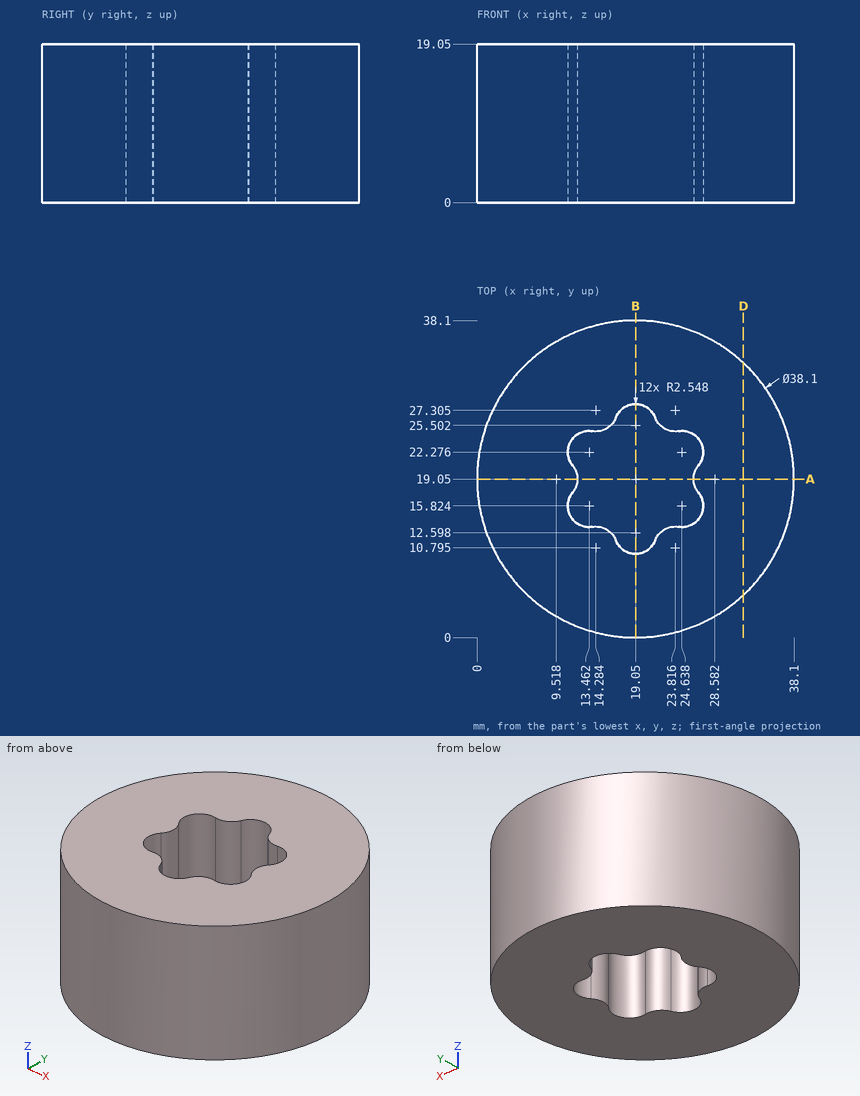
Input: dimensioned drawing with shaded views. Units: mm. Origin: part minimum x, y, z. Round coordinates to 2 decimals unless told otherwise and drop trailing zeros. Order: outer loops, then holes, each group sorted by start corner. A loop starts at its lowest first (then second) coordinate and runs counter-clockwise, first axis right, second up. Notation, with made-up numbers: (55, 76) -> (91, 76) arc R17 cw to (91, 96) -> close; hole circle Ø3 at (76, 78.25). An arc over 180 degrees is marked (long way). Put each result on its own line as item: value. Start each with the question number.
Q1. Section D-D on x = 32. Return the cut outline in (y, z), and give its area (3 significant figures).
Q2. First-contact query: pin 1 (1 mm diameter, centred on x = 30.5, z = 9.5, fed in from -Y); pin 2 (2 mm diameter, centred on x = 21, z = 11, fed in from -Y); pin 3 (8 mm diameter, centred on y = 33, z = 12.5, fed in from -X) (1 decimal); pin 4 (8 mm diameter, centred on x = 26.5, y = 17.5, fed in from +Z). Flat tips, straight axial feed; report the tip coordinate or a pass-through.
Q3. Line query: probe 1 along X at (y, z) = (19, 13.25) (1 decimal); probe 2 along Y at (x, z) = (24, 12.25) (1 decimal); probe 3 along Y at (x, z) = (14.5, 13). Output: solid intervals per line, ascending.
Q4. Section B-B on x = 19.05. Return the cut outline in (y, z).
Q5. Section A-A on y = 19.05. Return the cut outline in (x, z), and give its area (3 significant figures).
Ans:
1. outline: (5.08, 0) -> (33.02, 0) -> (33.02, 19.05) -> (5.08, 19.05) -> close
1. area: 532 mm2
2. pin 1: stops at y = 3.46
2. pin 2: stops at y = 0.02
2. pin 3: stops at x = 2.8
2. pin 4: stops at z = 19.05
3. probe 1: x = 0 to 12.1, 26 to 38.1
3. probe 2: y = 0.7 to 13.3, 24.8 to 37.4
3. probe 3: y = 0.55 to 13.33, 24.77 to 37.55
4. outline: (0, 0) -> (10.05, 0) -> (10.05, 19.05) -> (0, 19.05) -> close; (28.05, 0) -> (38.1, 0) -> (38.1, 19.05) -> (28.05, 19.05) -> close
5. outline: (0, 0) -> (12.07, 0) -> (12.07, 19.05) -> (0, 19.05) -> close; (26.03, 0) -> (38.1, 0) -> (38.1, 19.05) -> (26.03, 19.05) -> close
5. area: 460 mm2
